from build123d import *

# Parameters (mm, degrees)
SKETCH_1_R      = 1.75
SKETCH_1_W      = 40
SKETCH_1_H      = 20
EXTRUDE_1_DEPTH = 4


with BuildPart() as part:
    # 草图1 → 凸台-拉伸1 (new body)
    with BuildSketch(Plane(origin=(0, 0, 0), x_dir=(1, 0, 0), z_dir=(0, 1, 0))):
        with BuildLine():
            Line((-22, 13), (22, 13))
            ThreePointArc((22, 13), (25.535533906, 11.535533906), (27, 8))
            Line((27, 8), (27, -8))
            ThreePointArc((27, -8), (25.535533906, -11.535533906), (22, -13))
            Line((22, -13), (-22, -13))
            ThreePointArc((-22, -13), (-25.535533906, -11.535533906), (-27, -8))
            Line((-27, -8), (-27, 8))
            ThreePointArc((-27, 8), (-25.535533906, 11.535533906), (-22, 13))
        make_face()
        with Locations((-23, -8)):
            Circle(SKETCH_1_R, mode=Mode.SUBTRACT)
        with Locations((-23, 8)):
            Circle(SKETCH_1_R, mode=Mode.SUBTRACT)
        with Locations((23, 8)):
            Circle(SKETCH_1_R, mode=Mode.SUBTRACT)
        with Locations((23, -8)):
            Circle(SKETCH_1_R, mode=Mode.SUBTRACT)
        with Locations((0, -0.5)):
            Rectangle(SKETCH_1_W, SKETCH_1_H, mode=Mode.SUBTRACT)
    extrude(amount=EXTRUDE_1_DEPTH)


solid = part.part
Geometry: final body of the model. Coordinates: model frame, mm. A direction names the side the tool comes from. Give positions to 0.01 mm unless a question says otherwise; leave off trailing zeros. Loops run counter-clockwise (first coordinate to the right, second up) from the corner with the lowest first, then second, coordinate; pieces in that order, holes last. Notation, with made-up numbers: M 56,-11 L 96,-11 A18 cw 96,-6 Z; hole C 45,22 d9. An arc over 180 degrees is marked long. Put each result on its own line as item: value. Start each with the question number.
1) Cut plane A-A (x = 4.5). Output: boundary loops of the cut face in (y, z).
2) Access query for faces 1 (the flat face through (20, 2, 1)), 2 (the flat face through (-2, 0, -11)). Directions: +Z, -Z, +X, -X, +Y, -Y. A direction counts if a zero-diameter tool reaches every point of the face in a straight line with its end or side. Return the directions, or none.
3) Pull-direction query (X, two-part tool) for faces 3 (the cylindrical face through (26, 2, 11)), 4 (the cylindrical face through (21.25, 1.97, 7.92)), 5 (the cylindrical face through (-24.75, 1.97, -8.08)), 6 (the cylindrical face through (-25, 2, 12)); classes: pulls with the +X half, pulls with the -X half, needs draft (parallel to the pull), parting line crosses it, or undercut.
4) Cut plane B-B (y = 2.1). Output: boundary loops of the cut face in (x, z).
5) Contact query for a flat-ended pin moving along its axis: pin 1 (12 mm diameter, centred on x = -5.5, z = 8, fed in from -Y). Output: stop coordinate, or through.
6) Ray query, line 1 along X through (y, z) = (2, -8); line 2 along X through (y, z) = (0.75, 6); line 3 along Z through (x, y) = (23, 2.55). Return the intervals inside material, ascending.
7) Cut plane C-C (x = 23). Output: boundary loops of the cut face in (y, z).
Verdict:
1. outline: M 0,-13 L 4,-13 L 4,-9.5 L 0,-9.5 Z; M 0,10.5 L 4,10.5 L 4,13 L 0,13 Z
2. face 1: +Y, -Y
2. face 2: +Z, -Z, +X, -X, -Y
3. face 3: pulls with the +X half
3. face 4: undercut
3. face 5: undercut
3. face 6: pulls with the -X half
4. outline: M -27,-8 A5 ccw -22,-13 L 22,-13 A5 ccw 27,-8 L 27,8 A5 ccw 22,13 L -22,13 A5 ccw -27,8 Z; hole C -23,-8 d3.5; hole C -23,8 d3.5; hole M -20,-9.5 L 20,-9.5 L 20,10.5 L -20,10.5 Z; hole C 23,-8 d3.5; hole C 23,8 d3.5
5. pin 1: y = 0
6. line 1: -27 to -24.75, -21.25 to -20, 20 to 21.25, 24.75 to 27
6. line 2: -27 to -20, 20 to 27
6. line 3: -12.9 to -9.75, -6.25 to 6.25, 9.75 to 12.9
7. outline: M 0,-12.9 L 4,-12.9 L 4,-9.75 L 0,-9.75 Z; M 0,-6.25 L 4,-6.25 L 4,6.25 L 0,6.25 Z; M 0,9.75 L 4,9.75 L 4,12.9 L 0,12.9 Z
